Autodesk Inventor part; units mm, degrees
ref_plane "РабПлоскость1" through (0, 0, 150) normal (0, 0, 1) x (1, 0, 0)
ref_plane "YZ Plane" through (0, 0, 0) normal (1, 0, 0) x (0, 1, 0)
ref_plane "XZ Plane" through (0, 0, 0) normal (0, 1, 0) x (-1, 0, 0)
sketch "Эскиз1" plane through (0, 0, 0) normal (0, 0, 1) x (1, 0, 0)
  arc A0 (0, -35) -> (0, 35) centre (0, 0) ccw
  arc A1 (0, -45) -> (0, 45) centre (0, 0) ccw
  line L0 (0, 45) -> (0, 35)
  line L1 (0, -45) -> (0, -35)
  line L2 (0, -63) -> (0, 63)
revolve "Вращение1" add sketch "Эскиз1" angle 360 about axis through (0, -10, 0) along (0, 1, 0) contours A0 L0 A1 L1
ref_plane "РабПлоскость1" through (0, 0, 150) normal (0, 0, 1) x (1, 0, 0)
sketch "Эскиз2" plane through (0, 0, 150) normal (0, 0, 1) x (1, 0, 0)
  line L0 (-60, 0) -> (-60, 20)
  line L1 (-60, 20) -> (10, 20)
  line L2 (10, 20) -> (10, -36)
  line L3 (-10, 0) -> (-60, 0)
  line L4 (-10, 0) -> (-10, -36)
  line L5 (-10, -36) -> (10, -36)
  point P0 (0, 0)
extrude "Выдавливание1" cut sketch "Эскиз2" against normal blind 250
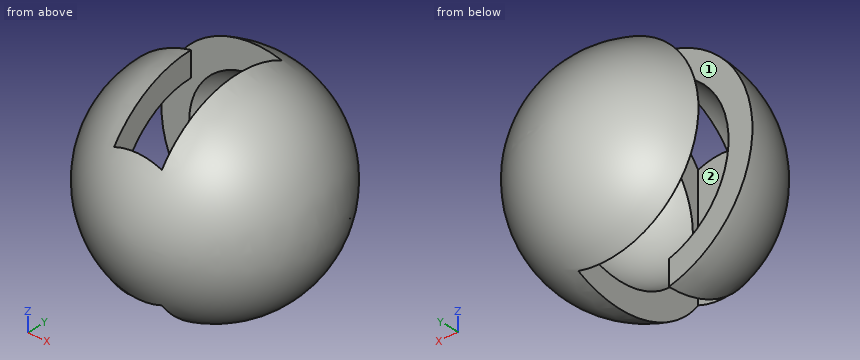
Geometry check sheet. Reference: the model listing, model coordinates, mm. Face numbers are marked on the shaded views. A direction names the side the tool comes from. Round coordinates to 2 decimals unless told otherwise and drop trailing zeros. Order: outer loops, then holes, each group sorted by start corner. A loop starts at its lowest first (then second) coordinate and runs counter-clockwise, first axis right, second up. Notation, with made-up numbers: M 35,-18.5 L 60,-18.5 A9 cw 60,-13.5 Z; hole C -0.75,7.25 d9. An arc over 180 degrees is marked long. Write item = value, one per line.
Q1. Scan lines: line 1 (Y direction, x = -14, z = -16.5); line 2 (Z direction, x = 23, y = 18); line 3 (Y direction, x = -2, z = 24.5). Record each from-to range of solid material in increasing order.
Answer block:
line_1 = -39.46 to -27.51, 27.51 to 39.46
line_2 = -34.23 to -19.29, 19.29 to 34.23
line_3 = -37.69 to -36, 24.91 to 37.69
Q2. Section check A-A (z = -30). Enter the section's corners in (x, y).
Answer block:
outline = M -33.54,0 A33.54 ccw -10,-32.02 L -10,-15 A18.03 cw -18.03,0 Z; M -26.93,20 L 10,20 L 10,15 A18.03 cw 10,-15 L 10,-32.02 A33.54 ccw long Z
Q3. Section check D-D (z = 21). Enter the section's corners in (x, y), plus the area to 3 significant figures.
Answer block:
outline = M -39.8,0 A39.8 ccw long -34.41,20 L -19.6,20 A28 cw long 10,-26.15 L 10,-36 L -10,-36 L -10,-26.15 A28 cw -28,0 Z
area = 2,090 mm^2
Q4. Set-up check for the marked faces 1 and 2: record each of +Z, -Z, +X, -X, +Y, -Y from which the full face is reachable in a straight line by a thin tool's end or side.
Answer block:
face_1 = +Z, -Z, -X
face_2 = +Z, -Z
Q5. Section check C-C (x = -13). Enter the section's corners in (y, z), plus the area to 3 significant figures.
Answer block:
outline = M 0,-43.08 L 0,-32.5 A32.5 cw 0,32.5 L 0,43.08 A43.08 ccw Z; M 20,-38.16 A43.08 ccw 20,38.16 L 20,25.61 A32.5 cw 20,-25.61 Z
area = 2,070 mm^2
Q6. Section check B-B (y = -25). Enter the section's corners in (x, z).
Answer block:
outline = M -10,-36.06 L -10,-22.36 A24.49 cw -10,22.36 L -10,36.06 A37.42 ccw Z; M 10,-36.06 A37.42 ccw 10,36.06 L 10,22.36 A24.49 cw 10,-22.36 Z
Q7. Depth check by flat-ended pin: pin 1 Ø2 at (x, z) = (22, 26) entering from -Y; pin 2 Ø25 at (x, z) = (-24.5, 8.5) entering from -Y; pin 3 Ø1 at (x, y) = (-28, -8.5) entering from +Z; pin 4 Ø22 at (x, z) = (-2, 5.5) entering from +Y. Enter the tip coordinate at first touch or a pass-through.
Answer block:
pin_1 = -30.53
pin_2 = -42.95
pin_3 = 34.61
pin_4 = 45
